The listing builds one solid part. Answer for the finished solid, in the listing's coordinates (mm). A direction names the side the tool comes from. Coordinates: 2 decimals unless noted, no trailing zeros. Write each loop counter-clockwise with the first axis right and the second up, starting at its lowest first coordinate (ties: lowest second). Pieces come first, ordered by that corner, then holes.
from build123d import *

# Parameters (mm, degrees)
EXTRUDE_1_DEPTH     = 52
SKETCH_2_R          = 26
CUT_EXTRUDE_1_DEPTH = 52


with BuildPart() as part:
    # 草图1 → 凸台-拉伸1 (new body)
    with BuildSketch(Plane.XY):
        Polygon((-37.84512636, 44.347033455), (206.15487364, 44.347033455), (291.15487364, 44.347033455), (291.15487364, -97.652966545), (292.65487364, -97.652966545), (292.65487364, 45.847033455), (-49.34512636, 45.847033455), (-49.34512636, 24.347033455), (-47.84512636, 24.347033455), (-47.84512636, 44.347033455), align=None)
    extrude(amount=EXTRUDE_1_DEPTH)

    # 草图2 → 切除-拉伸1 (cut)
    with BuildSketch(Plane.ZY.offset(-291.15487364)):
        with Locations((26, -97.652966545)):
            Circle(SKETCH_2_R)
    extrude(amount=-CUT_EXTRUDE_1_DEPTH, mode=Mode.SUBTRACT)


solid = part.part
1. A tool of negligible diameter and unlimited length cuts with its end or side. For faces 4 (the cylindrical face through (291.89, -71.66, 26.57)), 5 (the flat face through (119, 44.347, 26)), from which of +Z, -Z, +X, -X, +Y, -Y can it reach the whole face along a straight path? Write none if from no direction.
Results found:
face 4: +X, -X, -Y
face 5: +Z, -Z, -Y
2. Section C-C on x = 157 is taken. Give the vertices of the cut face in (y, z).
Results found:
outline: (44.35, 0) - (45.85, 0) - (45.85, 52) - (44.35, 52) - close
3. Section D-D on z = 5.5 is taken. Give the vertices of the cut face in (x, y).
Results found:
outline: (-49.35, 24.35) - (-47.85, 24.35) - (-47.85, 44.35) - (291.15, 44.35) - (291.15, -81.66) - (292.65, -81.66) - (292.65, 45.85) - (-49.35, 45.85) - close
4. Flat-ended cylindrical pins translate along their axes: P1, Ø12, axis at x = 94, z = 23, coming from the -Y side; P2, Ø12, axis at y = -73.5, z = 30.5, coming from the -X side; P3, Ø1.2, axis at x = -49, z = 28, coming from the -Y side. Find the tip coordinate at first contact, or state that the pin passes through.
Results found:
P1: stops at y = 44.35
P2: stops at x = 291.15
P3: stops at y = 24.35
5. Find the intervals of material crossed by L1, parallel to X at y = 40, z = 15.5; L2, parallel to Y at x = 226.5, z = 32.5; L3, parallel to X at y = -67, z = 23, in increasing order.
Results found:
L1: x = -49.35 to -47.85, 291.15 to 292.65
L2: y = 44.35 to 45.85
L3: x = 291.15 to 292.65
6. For a pull along X with two mould halves and no side action, classify faces 1 (the flat face through (292.655, -11, 26)), 2 (the flat face through (-47.845, 34, 26)), 3 (the flat face through (-49.345, 35, 26)) as pulls with the +X half, pulls with the -X half, needs draft (parallel to the pull), parting line crosses it, or undercut.
Results found:
face 1: pulls with the +X half
face 2: undercut
face 3: pulls with the -X half
7. Section A-A on z = 26 is taken. Give the vertices of the cut face in (x, y), then the cut area to 3 significant figures.
Results found:
outline: (-49.35, 24.35) - (-47.85, 24.35) - (-47.85, 44.35) - (291.15, 44.35) - (291.15, -71.65) - (292.65, -71.65) - (292.65, 45.85) - (-49.35, 45.85) - close
area: 717 mm2
8. Section B-B on y = -60.5 is taken. Give the vertices of the cut face in (x, z), then the cut area to 3 significant figures.
Results found:
outline: (291.15, 0) - (292.65, 0) - (292.65, 52) - (291.15, 52) - close
area: 78.0 mm2
